Can you work these out from the model? Positions are in its coordinate system, mm. Face numbers are marked on the shaded views. Give positions to 0.01 mm unless a question says otherwise; leave off trailing zeros. Order: outer loops, then holes, each group sorted by start corner. A loop starts at its lowest first (then second) coordinate and runs counter-clockwise, first axis right, second up. Notation, with made-up numbers: (65.25, 60) -> (101.25, 60) arc R15 ccw to (101.25, 85) -> close; hole circle Ø10 at (-26.75, 81). An arc over 180 degrees is marked (long way). Answer as CSV lines item,"result".
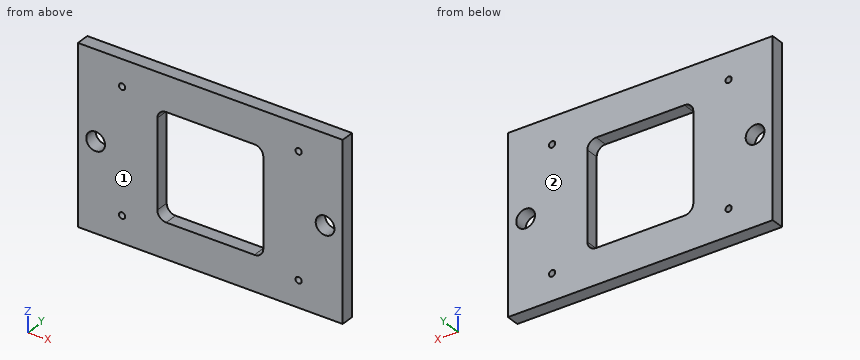
```python
from build123d import *

# Parameters (mm, degrees)
SKETCH1_W                        = 95.25
SKETCH1_H                        = 63.5
BOSS_EXTRUDE1_DEPTH              = 2.38125
CUT_EXTRUDE1_REACH               = 59.436
SKETCH2_W                        = 38.1
SKETCH2_H                        = 38.1
F_4_40_TAPPED_HOLE1_D            = 2.2606
F_17_64_0_26563_DIAMETER_HOLE1_D = 6.747002
FILLET1_R                        = 3.175
FILLET2_R                        = 3.175
FILLET3_R                        = 3.175
FILLET4_R                        = 3.175


with BuildPart() as part:
    # Sketch1 → Boss-Extrude1 (new, symmetric)
    with BuildSketch(Plane(origin=(0, 0, 0), x_dir=(1, 0, 0), z_dir=(0, 1, 0))):
        Rectangle(SKETCH1_W, SKETCH1_H)
    extrude(amount=BOSS_EXTRUDE1_DEPTH, both=True)

    # Sketch2 → Cut-Extrude1 (cut, up to next)
    with BuildSketch(Plane(origin=(0, 2.38125, 0), x_dir=(1, 0, 0), z_dir=(0, 1, 0)), mode=Mode.PRIVATE) as cut_extrude1_sk1:
        Rectangle(SKETCH2_W, SKETCH2_H)
    cut_extrude1_tool1 = extrude(cut_extrude1_sk1.sketch, amount=-CUT_EXTRUDE1_REACH, mode=Mode.PRIVATE) & part.part
    add(cut_extrude1_tool1.solids().sort_by_distance((0, 2.38125, 0))[0], mode=Mode.SUBTRACT)

    # #4-40 Tapped Hole1 (through all)
    with Locations(Plane(origin=(0, 2.38125, 0), x_dir=(1, 0, 0), z_dir=(0, 1, 0))):
        with Locations((-31.75, 22.225), (31.75, 22.225)):
            f_4_40_tapped_hole1 = Hole(F_4_40_TAPPED_HOLE1_D / 2)

    # Mirror1: #4-40 Tapped Hole1 across plane
    add(f_4_40_tapped_hole1.mirror(Plane.XY), mode=Mode.SUBTRACT)

    # 17/64 (0.26563) Diameter Hole1 (through all)
    with Locations(Plane(origin=(0, 2.38125, 0), x_dir=(1, 0, 0), z_dir=(0, 1, 0))):
        with Locations((-41.275, 0), (41.275, 0)):
            Hole(F_17_64_0_26563_DIAMETER_HOLE1_D / 2)

    # Fillet1
    fillet1_edges = [part.edges().sort_by_distance(p)[0] for p in [
        (-19.05, 0, -19.05),
    ]]
    fillet(fillet1_edges, radius=FILLET1_R)

    # Fillet2
    fillet2_edges = [part.edges().sort_by_distance(p)[0] for p in [
        (-19.05, 0, 19.05),
    ]]
    fillet(fillet2_edges, radius=FILLET2_R)

    # Fillet3
    fillet3_edges = [part.edges().sort_by_distance(p)[0] for p in [
        (19.05, 0, -19.05),
    ]]
    fillet(fillet3_edges, radius=FILLET3_R)

    # Fillet4
    fillet4_edges = [part.edges().sort_by_distance(p)[0] for p in [
        (19.05, 0, 19.05),
    ]]
    fillet(fillet4_edges, radius=FILLET4_R)


solid = part.part
```
Item 1: We'd pull the mould along Y, two halves only. Please class the marked faces 1 and 2: released by +Y, released by -Y, zero draft, split by the parting line, or undercut.
Numbers:
face 1,"released by -Y"
face 2,"released by +Y"
Item 2: Imagine slicing it at D-D, the plane x = -31.75. Please give me the cut outline in (y, z), then the cut area to 3 significant figures.
Numbers:
outline,"(-2.38, -31.75) -> (2.38, -31.75) -> (2.38, -23.36) -> (-2.38, -23.36) -> close; (-2.38, -21.09) -> (2.38, -21.09) -> (2.38, 21.09) -> (-2.38, 21.09) -> close; (-2.38, 23.36) -> (2.38, 23.36) -> (2.38, 31.75) -> (-2.38, 31.75) -> close"
area,"281 mm²"
Item 3: Imagine slicing it at B-B, the plane x = 2. Please give me the cut outline in (y, z), then the cut area to 3 significant figures.
Numbers:
outline,"(-2.38, -31.75) -> (2.38, -31.75) -> (2.38, -19.05) -> (-2.38, -19.05) -> close; (-2.38, 19.05) -> (2.38, 19.05) -> (2.38, 31.75) -> (-2.38, 31.75) -> close"
area,"121 mm²"
Item 4: For pin 1 (9 mm diameter, centred on x = -41.275, z = 0, fed in from -Y); pin 2 (1.8 mm diameter, centred on x = 31.75, z = 22.225, fed in from -Y), each with a flat end and sliding along its axis, tell me the tip position at first contact or that it passes through.
Numbers:
pin 1,"stops at y = -2.38"
pin 2,"passes through"
Item 5: Imagine slicing it at A-A, the plane z = 0. Give the number of separate pieces and of enclosed holes in the cut face, then the cut area to 3 significant figures.
Numbers:
separate pieces,"4"
enclosed holes,"0"
area,"208 mm²"
Item 6: Imagine slicing it at C-C, the plane z = -13. Please give me the cut outline in (x, y) (3 decimals).
Numbers:
outline,"(-47.625, -2.381) -> (-19.05, -2.381) -> (-19.05, 2.381) -> (-47.625, 2.381) -> close; (19.05, -2.381) -> (47.625, -2.381) -> (47.625, 2.381) -> (19.05, 2.381) -> close"
Item 7: Please list where these lines run through material, in increasing order: line 1 along Z through (x, y) = (31.75, 0.15); line 2 along Z through (x, y) = (15.5, -2.2); line 3 along X through (y, z) = (0.9, 4) (3 decimals).
Numbers:
line 1,"z = -31.75 to -23.36, -21.09 to 21.09, 23.36 to 31.75"
line 2,"z = -31.75 to -19.05, 19.05 to 31.75"
line 3,"x = -47.625 to -19.05, 19.05 to 47.625"
